Build history of the part. All positions in model axes, mm. A direction names the side the tool comes from. Round coordinates to 2 decimals unless told otherwise and drop trailing zeros. Write each loop counter-clockwise with the first axis right and the second up, starting at its lowest first coordinate (ties: lowest second). Pieces come first, ordered by that corner, then holes. Notation, with made-up numbers: M 22,-29 L 78,-29 A25 cw 78,-3 Z; hole C 47,76.25 d2. An arc over 180 degrees is marked long. Use a Markdown table: item, result.
from build123d import *

# Parameters (mm, degrees)
BOSS_EXTRUDE1_DEPTH = 50


with BuildPart() as part:
    # Sketch1 → Boss-Extrude1 (new body)
    with BuildSketch(Plane(origin=(0, 0, 0), x_dir=(1, 0, 0), z_dir=(0, 1, 0))):
        Polygon((3, 46.72), (0, 46.72), (0, 0), (0.000186337, -0.03343628), (3, 0), align=None)
        Polygon((3, 0), (0.000186337, -0.03343628), (0.000186337, -9.413789645), (-8.16140534, -11.826136958), (-33.586790943, -19.341198123), (-29.724787296, -19.341198123), (-7.554025616, -14.764008615), (3, -12.585113004), align=None)
    extrude(amount=BOSS_EXTRUDE1_DEPTH)


solid = part.part
Q1. Cut at B-B on z = -22. Give the cut face in (x, y).
Response values:
| item | result |
|---|---|
| outline | M 0,0 L 3,0 L 3,50 L 0,50 Z |
Q2. Drill centre lines: L1, parallel to X at y = 45, z = -20.5; L2, parallel to Z at x = -19.5, y = 26; L3, parallel to Z at x = -1.5, y = 4. Where is each one in solid material? Low to high.
Response values:
| item | result |
|---|---|
| L1 | x = 0 to 3 |
| L2 | z = 15.18 to 17.23 |
| L3 | z = 9.86 to 13.51 |
Q3. Drop flat-ended pins along their axis: P1, Ø4, axis at y = 20, z = -19.5, coming from the -X side; P2, Ø1.5, axis at x = -13.5, y = 16, coming from the +Z side; P3, Ø2, axis at x = -1.5, z = -0.5, coming from the +Y side; P4, Ø5, axis at x = -24, y = 20.5, coming from the -Z side. Give the stop position or say it passes through.
Response values:
| item | result |
|---|---|
| P1 | stops at x = 0 |
| P2 | stops at z = 16.15 |
| P3 | passes through |
| P4 | stops at z = 15.77 |
Q4. Cut at C-C on x = -5. Give the cut face in (y, z), and give its area (3 significant figures).
Response values:
| item | result |
|---|---|
| outline | M 0,10.89 L 50,10.89 L 50,14.24 L 0,14.24 Z |
| area | 167 mm2 |
Q5. Which spindle directions (+Z, -Z, +X, -X, +Y, -Y) get a long thin tool onto all of the face, cutting with end or side? Do faces 1 (the flat face through (0, 25, 5)), 2 (the flat face through (3, 25, -17)). Say none if no direction does.
Response values:
| item | result |
|---|---|
| face 1 | -Z, -X, +Y, -Y |
| face 2 | +Z, -Z, +X, +Y, -Y |
